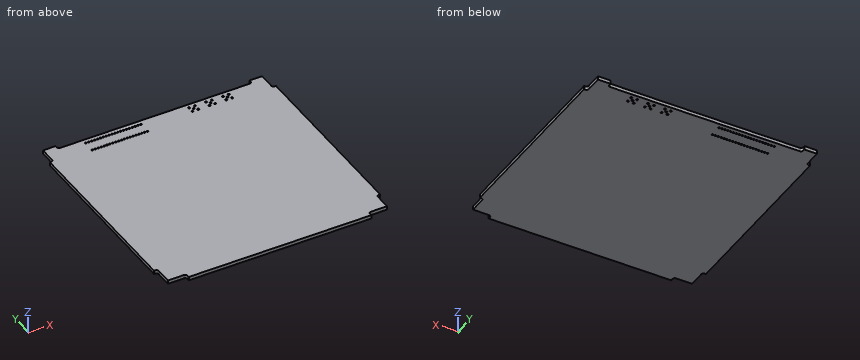
from build123d import *

# Parameters (mm, degrees)
BOSS_EXTRUDE1_DEPTH = 1.5875
SKETCH2_R           = 0.35
CUT_EXTRUDE1_DEPTH  = 71.728496069
CUT_EXTRUDE2_DEPTH  = 3.8375
FILLET2_R           = 1
SKETCH5_OUTSIDE_W   = 130.286
SKETCH5_OUTSIDE_H   = 130.286
SKETCH5_OUTSIDE_W_2 = 99
SKETCH5_OUTSIDE_H_2 = 100
CUT_EXTRUDE3_DEPTH  = 71.728496069
SKETCH8_W           = 85
SKETCH8_H           = 1.5875
CUT_EXTRUDE4_DEPTH  = 3.8375
FILLET1_R           = 1
SKETCH6_R           = 0.4
CUT_EXTRUDE5_DEPTH  = 71.375920287


with BuildPart() as part:
    # Sketch1 → Boss-Extrude1 (new body)
    with BuildSketch(Plane.XY):
        Polygon((40, 50), (-40, 50), (-40, 48), (-48, 48), (-48, 40), (-50, 40), (-50, -37.864895224), (-50, -40), (-48, -40), (-48, -48), (-40, -48), (-40, -50), (-37.864895224, -50), (40, -50), (40, -48), (48, -48), (48, -40), (50, -40), (50, 40), (48, 40), (48, 48), (40, 48), align=None)
    extrude(amount=BOSS_EXTRUDE1_DEPTH)

    # Sketch2 → Cut-Extrude1 (cut, through all)
    with BuildSketch(Plane.XY.offset(1.5875)):
        with Locations((-31.5, 44)):
            Circle(SKETCH2_R)
        with Locations((-30.23, 44)):
            Circle(SKETCH2_R)
        with Locations((-28.96, 44)):
            Circle(SKETCH2_R)
        with Locations((-27.69, 44)):
            Circle(SKETCH2_R)
        with Locations((-26.42, 44)):
            Circle(SKETCH2_R)
        with Locations((-25.15, 44)):
            Circle(SKETCH2_R)
        with Locations((-23.88, 44)):
            Circle(SKETCH2_R)
        with Locations((-22.61, 44)):
            Circle(SKETCH2_R)
        with Locations((-21.34, 44)):
            Circle(SKETCH2_R)
        with Locations((-20.07, 44)):
            Circle(SKETCH2_R)
        with Locations((-18.8, 44)):
            Circle(SKETCH2_R)
        with Locations((-17.53, 44)):
            Circle(SKETCH2_R)
        with Locations((-16.26, 44)):
            Circle(SKETCH2_R)
        with Locations((-14.99, 44)):
            Circle(SKETCH2_R)
        with Locations((-13.72, 44)):
            Circle(SKETCH2_R)
        with Locations((-12.45, 44)):
            Circle(SKETCH2_R)
        with Locations((-11.18, 44)):
            Circle(SKETCH2_R)
        with Locations((-9.91, 44)):
            Circle(SKETCH2_R)
        with Locations((-8.64, 44)):
            Circle(SKETCH2_R)
        with Locations((-7.37, 44)):
            Circle(SKETCH2_R)
        with Locations((-30.23, 38.92)):
            Circle(SKETCH2_R)
        with Locations((-28.96, 38.92)):
            Circle(SKETCH2_R)
        with Locations((-27.69, 38.92)):
            Circle(SKETCH2_R)
        with Locations((-26.42, 38.92)):
            Circle(SKETCH2_R)
        with Locations((-25.15, 38.92)):
            Circle(SKETCH2_R)
        with Locations((-23.88, 38.92)):
            Circle(SKETCH2_R)
        with Locations((-22.61, 38.92)):
            Circle(SKETCH2_R)
        with Locations((-21.34, 38.92)):
            Circle(SKETCH2_R)
        with Locations((-20.07, 38.92)):
            Circle(SKETCH2_R)
        with Locations((-18.8, 38.92)):
            Circle(SKETCH2_R)
        with Locations((-17.53, 38.92)):
            Circle(SKETCH2_R)
        with Locations((-16.26, 38.92)):
            Circle(SKETCH2_R)
        with Locations((-14.99, 38.92)):
            Circle(SKETCH2_R)
        with Locations((-13.72, 38.92)):
            Circle(SKETCH2_R)
        with Locations((-12.45, 38.92)):
            Circle(SKETCH2_R)
        with Locations((-11.18, 38.92)):
            Circle(SKETCH2_R)
        with Locations((-9.91, 38.92)):
            Circle(SKETCH2_R)
        with Locations((-8.64, 38.92)):
            Circle(SKETCH2_R)
        with Locations((-7.37, 38.92)):
            Circle(SKETCH2_R)
        with Locations((-31.5, 38.92)):
            Circle(SKETCH2_R)
    extrude(amount=-CUT_EXTRUDE1_DEPTH, mode=Mode.SUBTRACT)

    # Sketch3 → Cut-Extrude2 (cut)
    with BuildSketch(Plane(origin=(0, 50, 0), x_dir=(1, 0, 0), z_dir=(0, 1, 0))):
        Polygon((10.7, 0), (19.7, 0), (34.5, 0), (34.5, -1.5875), (19.7, -1.5875), (10.7, -1.5875), align=None)
    extrude(amount=-CUT_EXTRUDE2_DEPTH, mode=Mode.SUBTRACT)

    # Fillet2
    fillet2_edges = [part.edges().sort_by_distance(p)[0] for p in [
        (10.7, 46.1625, 0.79375),
        (34.5, 46.1625, 0.79375),
    ]]
    fillet(fillet2_edges, radius=FILLET2_R)

    # Sketch5 outside → Cut-Extrude3 (cut, through all)
    with BuildSketch(Plane(origin=(0, 0, 0), x_dir=(-1, 0, 0), z_dir=(0, 0, -1))):
        Rectangle(SKETCH5_OUTSIDE_W, SKETCH5_OUTSIDE_H)
        Rectangle(SKETCH5_OUTSIDE_W_2, SKETCH5_OUTSIDE_H_2, mode=Mode.SUBTRACT)
    extrude(amount=-CUT_EXTRUDE3_DEPTH, mode=Mode.SUBTRACT)

    # Sketch8 → Cut-Extrude4 (cut)
    with BuildSketch(Plane(origin=(0, 50, 0), x_dir=(1, 0, 0), z_dir=(0, 1, 0))):
        with Locations((0, -0.79375)):
            Rectangle(SKETCH8_W, SKETCH8_H)
    extrude(amount=-CUT_EXTRUDE4_DEPTH, mode=Mode.SUBTRACT)

    # Fillet1
    fillet1_edges = [part.edges().sort_by_distance(p)[0] for p in [
        (42.5, 46.1625, 0.79375),
        (-42.5, 46.1625, 0.79375),
        (-48, -40, 0.79375),
        (-48, 40, 0.79375),
        (48, 40, 0.79375),
        (48, -40, 0.79375),
        (40, -48, 0.79375),
        (-40, -48, 0.79375),
    ]]
    fillet(fillet1_edges, radius=FILLET1_R)

    # Sketch6 → Cut-Extrude5 (cut, through all)
    with BuildSketch(Plane.XY.offset(1.5875)):
        with Locations((29.94, 42.8925)):
            Circle(SKETCH6_R)
        with Locations((28.67, 44.1625)):
            Circle(SKETCH6_R)
        with Locations((31.21, 44.1625)):
            Circle(SKETCH6_R)
        with Locations((31.21, 41.6225)):
            Circle(SKETCH6_R)
        with Locations((28.67, 41.6225)):
            Circle(SKETCH6_R)
        with Locations((22.54, 42.8925)):
            Circle(SKETCH6_R)
        with Locations((21.27, 44.1625)):
            Circle(SKETCH6_R)
        with Locations((23.81, 44.1625)):
            Circle(SKETCH6_R)
        with Locations((23.81, 41.6225)):
            Circle(SKETCH6_R)
        with Locations((21.27, 41.6225)):
            Circle(SKETCH6_R)
        with Locations((15.14, 42.8925)):
            Circle(SKETCH6_R)
        with Locations((13.87, 44.1625)):
            Circle(SKETCH6_R)
        with Locations((16.41, 44.1625)):
            Circle(SKETCH6_R)
        with Locations((16.41, 41.6225)):
            Circle(SKETCH6_R)
        with Locations((13.87, 41.6225)):
            Circle(SKETCH6_R)
    extrude(amount=-CUT_EXTRUDE5_DEPTH, mode=Mode.SUBTRACT)


solid = part.part
Geometry: final body of the model. Coordinates: model frame, mm. Round coordinates to 2 decimals unless told otherwise and drop trailing zeros. Loops run counter-clockwise (first coordinate to the right, second up) from the corner with the lowest first, then second, coordinate; pieces in that order, holes last. Notation, with made-up numbers: M 31,-26 L 46,-26 A17 cw 46,2 Z; hole C -3.5,53 d9. An arc over 180 degrees is marked long. Put each result on its own line as item: value. Start each with the question number.
(1) Section query C-C (z = 1.3). State how many separate pieces and enclosed holes the cut face has, then the cut area to 3 significant figures.
(2) Section query A-A (x = -0.5). Return loops of the section in (y, z), then the cut area to 3 significant figures.
(3) Material intervals for line 1 along Y through (x, z) = (-13.72, 1.1); line 2 along Y through (x, z) = (14, 0.9); line 3 along Y through (x, z) = (1, 0.6), sorted ascending. Write a range as [from, to].
(4) Section query B-B (y = -43.5). Return loops of the section in (x, z), then the cut area to 3 significant figures.
(5) Contact query for flat-ended pins moving along their axis: pin 1 Ø0.9 at (y, z) = (47.5, 1) entering from -X; pin 2 Ø0.8 at (x, z) = (-43.5, 1) entering from -Y; pin 3 Ø0.5 at (x, z) = (-10, 1) entering from +Y. Output: stop coordinate, or through.
Findings below:
1. separate pieces: 1
1. enclosed holes: 55
1. area: 9,440 mm2
2. outline: M -50,0 L 46.16,0 L 46.16,1.59 L -50,1.59 Z
2. area: 153 mm2
3. line 1: y = [-50, 38.57], [39.27, 43.65], [44.35, 46.16]
3. line 2: y = [-50, 41.24], [42, 43.78], [44.54, 46.16]
3. line 3: y = [-50, 46.16]
4. outline: M -48,0 L 48,0 L 48,1.59 L -48,1.59 Z
4. area: 152 mm2
5. pin 1: stops at x = -48
5. pin 2: stops at y = -48
5. pin 3: stops at y = 46.16
